Read the model definition and answer for the solid it produces. Units are mm, in the model's axes. Face numbers are marked on the shaded views. Give positions to 0.01 mm unless a question says otherwise; leave off trailing zeros. Order: outer loops, then holes, each group sorted by start corner. A loop starts at its lowest first (then second) coordinate and runs counter-clockwise, first axis right, second up. Notation, with made-up numbers: M 79.5,27.5 L 98.5,27.5 A13 ccw 98.5,49.5 Z; hole C 48.25,24 d11. An arc over 180 degrees is marked long. One line per item, written item: value. Start each with the question number.
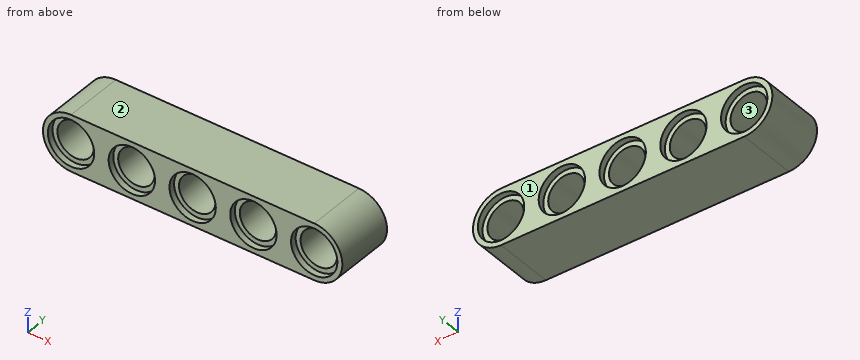
from build123d import *

# Parameters (mm, degrees)
BOSS_EXTRUDE3_DEPTH = 7.8
SKETCH2_R           = 2.4
CUT_EXTRUDE6_DEPTH  = 7.8
SKETCH3_R           = 3.05
CUT_EXTRUDE7_DEPTH  = 0.8
SKETCH4_R           = 3.05
CUT_EXTRUDE8_DEPTH  = 0.8


with BuildPart() as part:
    # Sketch1 → Boss-Extrude3 (new body)
    with BuildSketch(Plane(origin=(0, 0, 0), x_dir=(1, 0, 0), z_dir=(0, 1, 0))):
        with BuildLine():
            Line((-16, 3.7), (16, 3.7))
            ThreePointArc((16, 3.7), (19.7, 0), (16, -3.7))
            Line((16, -3.7), (0, -3.7))
            Line((0, -3.7), (-16, -3.7))
            ThreePointArc((-16, -3.7), (-19.7, 0), (-16, 3.7))
        make_face()
    extrude(amount=BOSS_EXTRUDE3_DEPTH)

    # Sketch2 → Cut-Extrude6 (cut)
    with BuildSketch(Plane(origin=(0, 7.8, 0), x_dir=(1, 0, 0), z_dir=(0, 1, 0))):
        Circle(SKETCH2_R)
        with Locations((8, 0)):
            Circle(SKETCH2_R)
        with Locations((16, 0)):
            Circle(SKETCH2_R)
        with Locations((-16, 0)):
            Circle(SKETCH2_R)
        with Locations((-8, 0)):
            Circle(SKETCH2_R)
    extrude(amount=-CUT_EXTRUDE6_DEPTH, mode=Mode.SUBTRACT)

    # Sketch3 → Cut-Extrude7 (cut)
    with BuildSketch(Plane(origin=(0, 7.8, 0), x_dir=(1, 0, 0), z_dir=(0, 1, 0))):
        Circle(SKETCH3_R)
        with Locations((8, 0)):
            Circle(SKETCH3_R)
        with Locations((16, 0)):
            Circle(SKETCH3_R)
        with Locations((-16, 0)):
            Circle(SKETCH3_R)
        with Locations((-8, 0)):
            Circle(SKETCH3_R)
    extrude(amount=-CUT_EXTRUDE7_DEPTH, mode=Mode.SUBTRACT)

    # Sketch4 → Cut-Extrude8 (cut)
    with BuildSketch(Plane.XZ):
        Circle(SKETCH4_R)
        with Locations((8, 0)):
            Circle(SKETCH4_R)
        with Locations((16, 0)):
            Circle(SKETCH4_R)
        with Locations((-16, 0)):
            Circle(SKETCH4_R)
        with Locations((-8, 0)):
            Circle(SKETCH4_R)
    extrude(amount=-CUT_EXTRUDE8_DEPTH, mode=Mode.SUBTRACT)


solid = part.part
Q1. Determine the mould class of the marked faces 1, 2 and 3 for opening direction Z: released by +Z, released by -Z, zero draft, split by the parting line, or undercut.
Q2. Find section B-B, the plane y = 4.25. Give the vertices of the cut face in (x, z), then the cut area to 3 significant figures.
Q3. Find section D-D, the plane x = 16.5. Give the vertices of the cut face in (y, z).
Q4. Consider probe 1 along X at (y, z) = (7.4, 0); probe 2 along Z at (x, y) = (16, 6); probe 3 along X at (y, z) = (3.75, -1.75). Determine where each line is inside the solid, lowest interval first.
Q5. Find section C-C, the plane z = 0. State how many separate pieces and enclosed holes the cut face has, then the cut area to 3 significant figures.
Q6. Each of these flat-tipped pins is pushed along its axis until it touches: pin 1 (3 mm diameter, centred on x = -16, z = 1, fed in from +Y); pin 2 (3.5 mm diameter, centred on x = 0, z = 0, fed in from -Y); pin 3 (3 mm diameter, centred on x = 14.5, z = 0, fed in from -Y). Where does it stop, or does it pass through?
Q7. Find section A-A, the plane x = -8. Give the vertices of the cut face in (y, z), then the cut area to 3 significant figures.
Evaluation:
1. face 1: zero draft
1. face 2: released by +Z
1. face 3: undercut
2. outline: M -16,-3.7 L 16,-3.7 A3.7 ccw 16,3.7 L -16,3.7 A3.7 ccw Z; hole C -16,0 d4.8; hole C -8,0 d4.8; hole C 0,0 d4.8; hole C 8,0 d4.8; hole C 16,0 d4.8
2. area: 189 mm2
3. outline: M 0,-3.67 L 7.8,-3.67 L 7.8,-3.01 L 7,-3.01 L 7,-2.35 L 0.8,-2.35 L 0.8,-3.01 L 0,-3.01 Z; M 0,3.01 L 0.8,3.01 L 0.8,2.35 L 7,2.35 L 7,3.01 L 7.8,3.01 L 7.8,3.67 L 0,3.67 Z
4. probe 1: -19.7 to -19.05, -12.95 to -11.05, -4.95 to -3.05, 3.05 to 4.95, 11.05 to 12.95, 19.05 to 19.7
4. probe 2: -3.7 to -2.4, 2.4 to 3.7
4. probe 3: -19.26 to -17.64, -14.36 to -9.64, -6.36 to -1.64, 1.64 to 6.36, 9.64 to 14.36, 17.64 to 19.26
5. separate pieces: 6
5. enclosed holes: 0
5. area: 110 mm2
6. pin 1: y = 7
6. pin 2: through
6. pin 3: y = 0.8
7. outline: M 0,-3.7 L 7.8,-3.7 L 7.8,-3.05 L 7,-3.05 L 7,-2.4 L 0.8,-2.4 L 0.8,-3.05 L 0,-3.05 Z; M 0,3.05 L 0.8,3.05 L 0.8,2.4 L 7,2.4 L 7,3.05 L 7.8,3.05 L 7.8,3.7 L 0,3.7 Z
7. area: 18.2 mm2
